For this review, use the dimensioned drawing (mm, ordinates from the lowest corner) and the shaded views. A direction names the side the tool comes from. Round coordinates to 2 decimals unless told otherwise and drop trailing zeros. Write each loop counter-clockwise with the first axis right and the second up, starting at its lowest first coordinate (ties: lowest second). Pieces come first, ordered by that corner, then holes. Notation, with made-up numbers: (82, 17.5) -> (135, 17.5) arc R16 ccw to (135, 31.5) -> close; hole circle Ø11 at (-36.5, 7). An arc over 180 degrees is marked (long way). Answer as CSV lines item,"result". Start each with the question number.
Item 1: Machinability: for the marked faces 4 and 5, which of the approach directions +Z, -Z, +X, -X, +Y, -Y give a long, thin tool a straight path to every point of the face, cutting with its end or side? Answer none if there is none.
Item 2: Wall thickness on probe 1 along X at (y, z) = (2, 38.25); probe 2 along Z at (x, y) = (9, 1); probe 3 along X at (y, z) = (2, 24): over which ranges is each line inside the solid? List them lowest first. Write a range as from..to.
Item 3: For pin 1 Ø5.5 at (x, z) = (19.5, 3.5) entering from +Y; pin 2 Ø10.5 at (x, z) = (20, 25.5) entering from +Y; pin 3 Ø2 at (x, z) = (9.75, 38.25) entering from +Y; pin 4 Ø3 at (x, y) = (27, 32) entering from +Z, all flat-tipped, find the tip position at first contact; note any pin that passes through.
Item 4: Mouldability with a two-part tool opening along X and no side actions: class the marked faces 1, 2 and 3 as +X half, -X half, draft (parallel to the pull), parting line (faces both ways), or undercut.
Item 5: Take a section at A-A on x = 25.25. Give the boundary of the cut face in (y, z), then the cut area to 3 significant figures.
Item 6: Take a section at C-C on z = 2.5. Give the boundary of the cut face in (x, y).
Item 7: Take a section at B-B on y = 41.5. Give the boundary of the cut face in (x, z), then the cut area to 3 significant figures.
Item 8: Take a section at D-D on x = 15. Give the boundary of the cut face in (y, z), then the cut area to 3 significant figures.
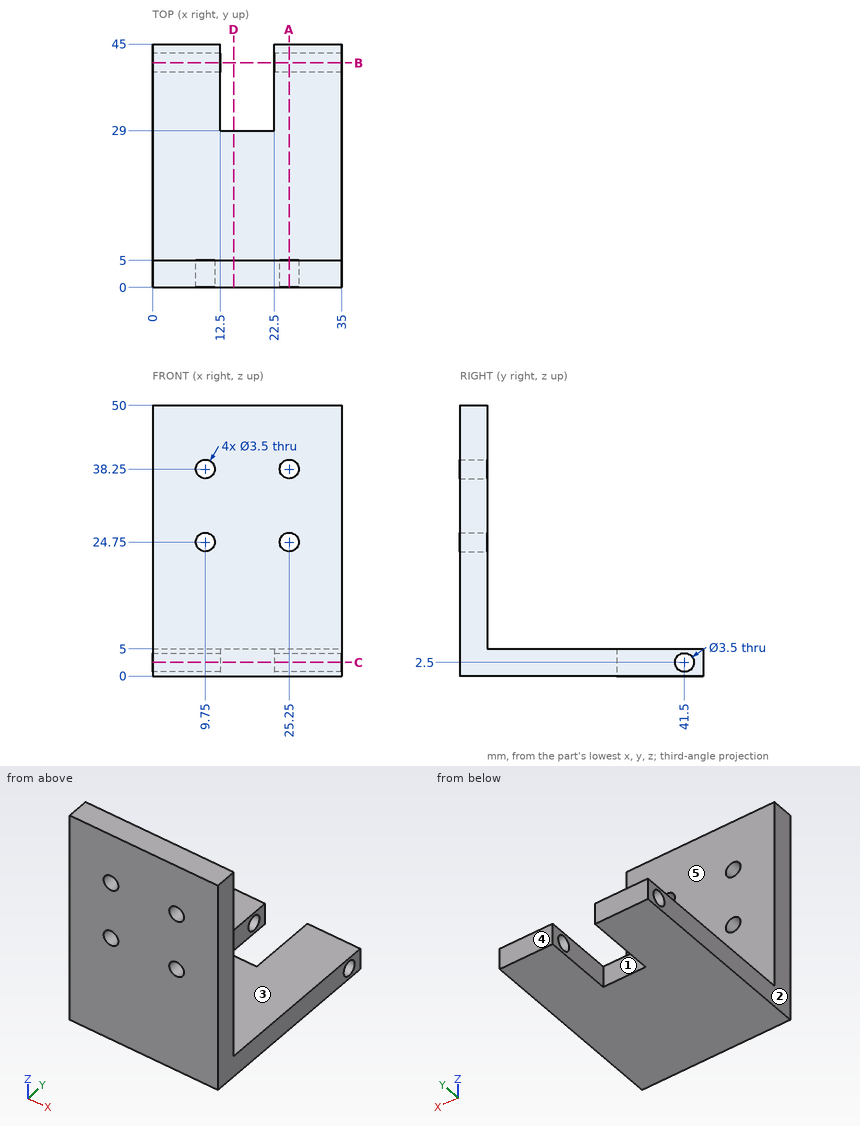
Output values:
1,face 4,"+Z, -Z, +X, -X, +Y"
1,face 5,"+Z, +X, -X, +Y"
2,probe 1,"x = 0..8, 11.5..23.5, 27..35"
2,probe 2,"z = 0..23.17, 26.33..36.67, 39.83..50"
2,probe 3,"x = 0..8.17, 11.33..23.67, 26.83..35"
3,pin 1,"stops at y = 29"
3,pin 2,"stops at y = 5"
3,pin 3,"passes through"
3,pin 4,"stops at z = 5"
4,face 1,"undercut"
4,face 2,"-X half"
4,face 3,"draft"
5,outline,"(0, 0) -> (45, 0) -> (45, 5) -> (5, 5) -> (5, 23) -> (0, 23) -> close; (0, 26.5) -> (5, 26.5) -> (5, 36.5) -> (0, 36.5) -> close; (0, 40) -> (5, 40) -> (5, 50) -> (0, 50) -> close; hole circle Ø3.5 at (41.5, 2.5)"
5,area,"405 mm^2"
6,outline,"(0, 0) -> (35, 0) -> (35, 39.75) -> (22.5, 39.75) -> (22.5, 29) -> (12.5, 29) -> (12.5, 39.75) -> (0, 39.75) -> close; (0, 43.25) -> (12.5, 43.25) -> (12.5, 45) -> (0, 45) -> close; (22.5, 43.25) -> (35, 43.25) -> (35, 45) -> (22.5, 45) -> close"
7,outline,"(0, 0) -> (12.5, 0) -> (12.5, 0.75) -> (0, 0.75) -> close; (0, 4.25) -> (12.5, 4.25) -> (12.5, 5) -> (0, 5) -> close; (22.5, 0) -> (35, 0) -> (35, 0.75) -> (22.5, 0.75) -> close; (22.5, 4.25) -> (35, 4.25) -> (35, 5) -> (22.5, 5) -> close"
7,area,"37.5 mm^2"
8,outline,"(0, 0) -> (29, 0) -> (29, 5) -> (5, 5) -> (5, 50) -> (0, 50) -> close"
8,area,"370 mm^2"
